CAD build for the part. Positions are in the model's coordinates, mm. A direction names the side the tool comes from. Give positions to 0.01 mm unless a question says otherwise; leave off trailing zeros. Loops run counter-clockwise (first coordinate to the right, second up) from the corner with the lowest first, then second, coordinate; pieces in that order, holes last. Notation, with made-up numbers: (84, 25) -> (97, 25) arc R33 ccw to (97, 58) -> close; hole circle Ø7 at (-26, 29.5). An arc over 180 degrees is marked (long way). Use one line per item in the form item = value.
```python
from build123d import *

# Parameters (mm, degrees)
F1_R      = 5.5
F2_DEPTH  = 10
F3_DEPTH  = 10
F5_DEPTH  = 10
F6_DEPTH  = 6
F7_DEPTH  = 10
F8_DEPTH  = 1
F9_DEPTH  = 1
F10_W     = 1
F10_H     = 3
F11_DEPTH = 10
F12_DEPTH = 8
F14_DEPTH = 1


with BuildPart() as f2:
    # F1 (on Top) → F2 (new body)
    with BuildSketch(Plane.XY):
        with Locations((23.6550478793, 2.625)):
            Circle(F1_R)
    extrude(amount=F2_DEPTH)

    # F0 (on Top) → F3 (cut)
    with BuildSketch(Plane.XY):
        with BuildLine():
            ThreePointArc((28.1550478793, 2.625), (27.733432921, 0.7232178222), (26.5475921229, -0.822199994))
            Line((26.5475921229, -0.822199994), (28.8864416499, -3.6095323204))
            Line((28.8864416499, -3.6095323204), (49.6550478793, -10.4956166668))
            Line((49.6550478793, -10.4956166668), (49.6550478793, 2.625))
            Line((49.6550478793, 2.625), (28.1550478793, 2.625))
        make_face()
        with BuildLine():
            Line((28.8864416499, 8.8595323204), (26.5475921229, 6.072199994))
            ThreePointArc((26.5475921229, 6.072199994), (27.733432921, 4.5267821778), (28.1550478793, 2.625))
            Line((28.1550478793, 2.625), (49.6550478793, 2.625))
            Line((49.6550478793, 2.625), (49.6550478793, 15.7456166668))
            Line((49.6550478793, 15.7456166668), (28.8864416499, 8.8595323204))
        make_face()
        with BuildLine():
            Line((23.6550478793, 2.625), (23.6550478793, -1.875))
            ThreePointArc((23.6550478793, -1.875), (25.1941385243, -1.6036167935), (26.5475921229, -0.822199994))
            Line((26.5475921229, -0.822199994), (23.6550478793, 2.625))
        make_face()
        with BuildLine():
            ThreePointArc((20, 5.25), (19.1550478793, 2.625), (20, 0))
            ThreePointArc((20, 0), (20.4453712418, -0.5290411987), (20.9665447643, -0.9835940476))
            Line((20.9665447643, -0.9835940476), (23.6550478793, -1.875))
            Line((23.6550478793, -1.875), (23.6550478793, 2.625))
            Line((23.6550478793, 2.625), (23.6550478793, 7.125))
            Line((23.6550478793, 7.125), (20.9665447643, 6.2335940476))
            ThreePointArc((20.9665447643, 6.2335940476), (20.4453712418, 5.7790411987), (20, 5.25))
        make_face()
        with BuildLine():
            ThreePointArc((26.5475921229, 6.072199994), (25.1941385243, 6.8536167935), (23.6550478793, 7.125))
            Line((23.6550478793, 7.125), (23.6550478793, 2.625))
            Line((23.6550478793, 2.625), (26.5475921229, 6.072199994))
        make_face()
        with BuildLine():
            Line((26.5475921229, 6.072199994), (23.6550478793, 2.625))
            Line((23.6550478793, 2.625), (28.1550478793, 2.625))
            ThreePointArc((28.1550478793, 2.625), (27.733432921, 4.5267821778), (26.5475921229, 6.072199994))
        make_face()
        with BuildLine():
            Line((23.6550478793, 2.625), (26.5475921229, -0.822199994))
            ThreePointArc((26.5475921229, -0.822199994), (27.733432921, 0.7232178222), (28.1550478793, 2.625))
            Line((28.1550478793, 2.625), (23.6550478793, 2.625))
        make_face()
        with BuildLine():
            Line((23.6550478793, -1.875), (20.9665447643, -0.9835940476))
            ThreePointArc((20.9665447643, -0.9835940476), (22.2388334206, -1.6463389712), (23.6550478793, -1.875))
        make_face()
        with BuildLine():
            ThreePointArc((23.6550478793, 7.125), (22.2388334206, 6.8963389712), (20.9665447643, 6.2335940476))
            Line((20.9665447643, 6.2335940476), (23.6550478793, 7.125))
        make_face()
    extrude(amount=F3_DEPTH, mode=Mode.SUBTRACT)

    # F4 (on Top) → F5 (join)
    with BuildSketch(Plane.XY):
        Polygon((0, 5.25), (18, 5.25), (19.0219422369, 5.5888373954), (20.506438149, 7.1345739007), (17.8385406763, 6.25), (0, 6.25), align=None)
        Polygon((19.0219422369, -0.3388373954), (18, 0), (0, 0), (0, -1), (17.8385406763, -1), (20.506438149, -1.8845739007), align=None)
    extrude(amount=F5_DEPTH)

    # F4 (on Top) → F6 (cut)
    with BuildSketch(Plane.XY):
        Polygon((0, 5.25), (18, 5.25), (19.0219422369, 5.5888373954), (20.506438149, 7.1345739007), (17.8385406763, 6.25), (0, 6.25), align=None)
        Polygon((19.0219422369, -0.3388373954), (18, 0), (0, 0), (0, -1), (17.8385406763, -1), (20.506438149, -1.8845739007), align=None)
    extrude(amount=F6_DEPTH, mode=Mode.SUBTRACT)

    # F0 (on Top) → F7 (cut)
    with BuildSketch(Plane.XY):
        with BuildLine():
            Line((0, 5.25), (0, 0))
            Line((0, 0), (18, 0))
            Line((18, 0), (20, 0))
            ThreePointArc((20, 0), (19.1550478793, 2.625), (20, 5.25))
            Line((20, 5.25), (18, 5.25))
            Line((18, 5.25), (0, 5.25))
        make_face()
        with BuildLine():
            Line((20, 0), (18, 0))
            Line((18, 0), (20.9665447643, -0.9835940476))
            ThreePointArc((20.9665447643, -0.9835940476), (20.4453712418, -0.5290411987), (20, 0))
        make_face()
        with BuildLine():
            Line((20.9665447643, 6.2335940476), (18, 5.25))
            Line((18, 5.25), (20, 5.25))
            ThreePointArc((20, 5.25), (20.4453712418, 5.7790411987), (20.9665447643, 6.2335940476))
        make_face()
    extrude(amount=F7_DEPTH, mode=Mode.SUBTRACT)

    # F1 (on Top) → F8 (join)
    with BuildSketch(Plane.XY):
        with Locations((23.6550478793, 2.625)):
            Circle(F1_R)
    extrude(amount=F8_DEPTH)

    # F0 (on Top) → F9 (cut)
    with BuildSketch(Plane.XY):
        with BuildLine():
            Line((0, 5.25), (0, 0))
            Line((0, 0), (18, 0))
            Line((18, 0), (20, 0))
            ThreePointArc((20, 0), (19.1550478793, 2.625), (20, 5.25))
            Line((20, 5.25), (18, 5.25))
            Line((18, 5.25), (0, 5.25))
        make_face()
        with BuildLine():
            ThreePointArc((28.1550478793, 2.625), (27.733432921, 0.7232178222), (26.5475921229, -0.822199994))
            Line((26.5475921229, -0.822199994), (28.8864416499, -3.6095323204))
            Line((28.8864416499, -3.6095323204), (49.6550478793, -10.4956166668))
            Line((49.6550478793, -10.4956166668), (49.6550478793, 2.625))
            Line((49.6550478793, 2.625), (28.1550478793, 2.625))
        make_face()
        with BuildLine():
            Line((28.8864416499, 8.8595323204), (26.5475921229, 6.072199994))
            ThreePointArc((26.5475921229, 6.072199994), (27.733432921, 4.5267821778), (28.1550478793, 2.625))
            Line((28.1550478793, 2.625), (49.6550478793, 2.625))
            Line((49.6550478793, 2.625), (49.6550478793, 15.7456166668))
            Line((49.6550478793, 15.7456166668), (28.8864416499, 8.8595323204))
        make_face()
    extrude(amount=F9_DEPTH, mode=Mode.SUBTRACT)

    # F10 (on Top) → F11 (join)
    with BuildSketch(Plane.XY):
        Polygon((23.4857258463, 8.122393023), (25.5996504067, 7.7697566522), (49.6550478793, 15.7456166668), (49.6550478793, 5.625), (50.6550478793, 5.625), (50.6550478793, 17.1307126516), align=None)
        Polygon((50.6550478793, -0.375), (49.6550478793, -0.375), (49.6550478793, -10.4956166668), (25.5996504067, -2.5197566522), (23.4857258463, -2.872393023), (50.6550478793, -11.8807126516), align=None)
        with Locations((50.1550478793, 1.125)):
            Rectangle(F10_W, F10_H)
        with Locations((50.1550478793, 4.125)):
            Rectangle(F10_W, F10_H)
    extrude(amount=F11_DEPTH)

    # F10 (on Top) → F12 (cut)
    with BuildSketch(Plane.XY):
        Polygon((23.4857258463, 8.122393023), (25.5996504067, 7.7697566522), (49.6550478793, 15.7456166668), (49.6550478793, 5.625), (50.6550478793, 5.625), (50.6550478793, 17.1307126516), align=None)
        Polygon((50.6550478793, -0.375), (49.6550478793, -0.375), (49.6550478793, -10.4956166668), (25.5996504067, -2.5197566522), (23.4857258463, -2.872393023), (50.6550478793, -11.8807126516), align=None)
    extrude(amount=F12_DEPTH, mode=Mode.SUBTRACT)

    # F13 (on face) → F14 (cut)
    with BuildSketch(Plane.YZ.offset(50.6550478793)):
        with BuildLine():
            ThreePointArc((2.625, 4.7), (3.5442388155, 5.0807611845), (3.925, 6))
            ThreePointArc((3.925, 6), (3.5442388155, 6.9192388155), (2.625, 7.3))
            Line((2.625, 7.3), (2.625, 4.7))
        make_face()
        with BuildLine():
            ThreePointArc((3.925, 2), (3.5442388155, 2.9192388155), (2.625, 3.3))
            Line((2.625, 3.3), (2.625, 0.7))
            ThreePointArc((2.625, 0.7), (3.5442388155, 1.0807611845), (3.925, 2))
        make_face()
        with BuildLine():
            Line((2.625, 0.7), (2.625, 3.3))
            ThreePointArc((2.625, 3.3), (1.325, 2), (2.625, 0.7))
        make_face()
        with BuildLine():
            Line((2.625, 4.7), (2.625, 7.3))
            ThreePointArc((2.625, 7.3), (1.325, 6), (2.625, 4.7))
        make_face()
    extrude(amount=-F14_DEPTH, mode=Mode.SUBTRACT)


solid = f2.part
```
1. Cut at B-B, the plane z = 9. Write the cut outline in (x, y) (3 decimals), then the cut area to 3 significant figures.
Result sheet:
outline = (0, -1) -> (17.839, -1) -> (20.506, -1.885) arc R5.5 ccw to (23.486, -2.872) -> (50.655, -11.881) -> (50.655, 17.131) -> (23.486, 8.122) arc R5.5 ccw to (20.506, 7.135) -> (17.839, 6.25) -> (0, 6.25) -> (0, 5.25) -> (18, 5.25) -> (20.967, 6.234) arc R4.5 cw to (26.548, 6.072) -> (27.19, 6.838) arc R5.5 ccw to (25.6, 7.77) -> (49.655, 15.746) -> (49.655, -10.496) -> (25.6, -2.52) arc R5.5 ccw to (27.19, -1.588) -> (26.548, -0.822) arc R4.5 cw to (20.967, -0.984) -> (18, 0) -> (0, 0) -> close
area = 136 mm^2
2. Drill centre lines: line 1 (Y direction, x = 2, z = 7.5); line 2 (Y direction, x = 34, z = 9) (3 decimals); line 3 (X direction, y = 5, z = 6.5). Where is each one in solid material? Low to high.
Result sheet:
line_1 = -1 to 0, 5.25 to 6.25
line_2 = -6.359 to -5.305, 10.555 to 11.609
line_3 = 49.66 to 50.66
3. Cut at A-A, the plane x = 5. Write the cut outline in (y, z), then the cut area to 3 significant figures.
Result sheet:
outline = (-1, 6) -> (0, 6) -> (0, 10) -> (-1, 10) -> close; (5.25, 6) -> (6.25, 6) -> (6.25, 10) -> (5.25, 10) -> close
area = 8.00 mm^2
4. Tool access for faces 1 (the flat face through (0, -0.5, 8)), 2 (the flat face through (24.53, 7.95, 3.94)), 3 (the flat face through (19.2, 6.7, 8)), 4 (the flat face through (19.77, -1.12, 3.46)), 5 (the flat face through (37.796, -6.564, 8.986)): list every direction of +Z, -Z, +X, -X, +Y, -Y with a clear straight run to the whole face (end or side of a thin tool).
Result sheet:
face_1 = +Z, -Z, -X, +Y, -Y
face_2 = -Z, +X, +Y
face_3 = +Z, -Z, -X, +Y
face_4 = -X, -Y
face_5 = +Z, -Z
5. Mould opens along X. For faces 6 (the cylindrical face through (26.42, -2.13, 4.93)), 7 (the flat face through (10.1, -0.5, 6)), 8 (the flat face through (36.88, -7.313, 8.986)) say: pulls with the +X half, pulls with the -X half, needs draft (parallel to the pull), parting line crosses it, or undercut.
Result sheet:
face_6 = undercut
face_7 = needs draft
face_8 = pulls with the -X half
6. Cut at C-C, the plane y = 11.25. Write the cut outline in (x, z).
Result sheet:
outline = (32.92, 8) -> (36.1, 8) -> (36.1, 10) -> (32.92, 10) -> close; (49.66, 8) -> (50.66, 8) -> (50.66, 10) -> (49.66, 10) -> close
7. Drop flat-ended pins along their axis: P1, Ø7, axis at x = 23, y = 1, coming from the +Z side; P2, Ø2, axis at x = 6.5, z = 7.5, coming from the -Y side; P3, Ø0.5, axis at x = 50.5, z = 5.5, coming from the +Y side (3 decimals); P4, Ø4.5, axis at x = 12.5, z = 7, coming from the +Y side. Give the stop position or say it passes through.
Result sheet:
P1 = 10
P2 = -1
P3 = 5.625
P4 = 6.25
